```python
from build123d import *

# Parameters (mm, degrees)
F0_R     = 57.15
F0_R_2   = 27.432
F1_DEPTH = 27.94
F2_R     = 35.052
F2_R_2   = 23.495
F3_DEPTH = 5.08
F5_D     = 3.7973


with BuildPart() as f1:
    # F0 (on Top) → F1 (new body)
    with BuildSketch(Plane.XY):
        Circle(F0_R)
        Circle(F0_R_2, mode=Mode.SUBTRACT)
    extrude(amount=F1_DEPTH)

    # F2 (on face) → F3 (join)
    with BuildSketch(Plane.XY.offset(27.94)):
        Circle(F2_R)
        Circle(F2_R_2, mode=Mode.SUBTRACT)
    extrude(amount=F3_DEPTH)

    # F5 (through all)
    with Locations(Plane.XY.offset(27.94)):
        with Locations((0, -53.34), (46.1937950379, -26.67), (46.1937950379, 26.67), (0, 53.34), (-46.1937950379, 26.67), (-46.1937950379, -26.67)):
            Hole(F5_D / 2)


solid = f1.part
```
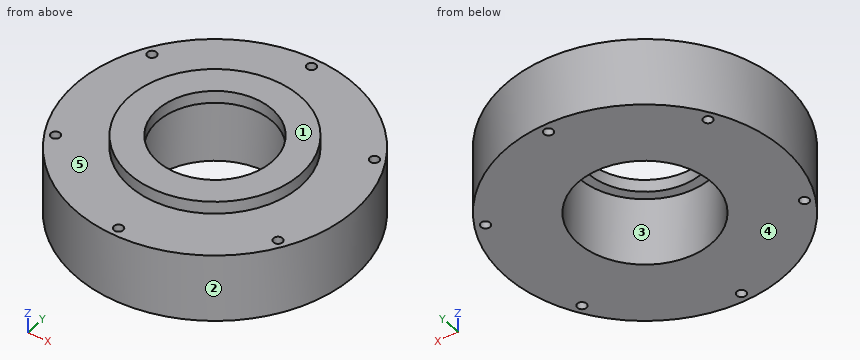
Can you work these out from the model? Positions are in its coordinate system, mm. Face numbers are marked on the shaded views. A direction names the side the tool comes from. Coordinates: 2 decimals unless noted, no trailing zeros. Loops run counter-clockwise (first coordinate to the right, second up) from the corner with the lowest first, then second, coordinate; pieces in that order, holes last.
1) Imagine slicing it at D-D on x = 15. List the corners of the cut face in (y, z) for me.
2) Thinking about a two-plate mould opening in X: for the marked faces 1, 2 and 3, which applies, pulls with the +X half, pulls with the -X half, needs draft (parallel to the pull), parting line crosses it, or undercut?
3) I need wall thicknesses on probe 1 along Y at (x, z) = (0, 19); probe 2 along Y at (x, z) = (0, 31.5) (3 decimals); probe 3 along Z at (x, y) = (-50, 22). Which ranges of each line are inside material? Lowest first, please.
4) Which directions (+Z, -Z, +X, -X, +Y, -Y) give clear straight access to the entire face, cutting with the end or side of a thin tool? Please do the marked faces 4 and 5.
5) Imagine slicing it at B-B on y = 0. List the corners of the cut face in (x, z) for me (3 decimals).
6) Imagine slicing it at A-A on x = 0. List the corners of the cut face in (y, z) for me (3 decimals), plus the area to 3 significant figures.
7) Imagine slicing it at C-C on z = 12. List the corners of the cut face in (x, y) for me.
8) For pin 1 (3 mm diameter, centred on x = 2, z = 9, fed in from -Y); pin 2 (4 mm diameter, centred on x = -32, z = 10, fed in from -Y); pin 3 (8 mm diameter, centred on x = 28.5, z = 15.5, fed in from +Y); pin 4 (2.5 mm diameter, centred on x = -46.19, y = 26.67, fed in from +Z), each with a flat end and sliding along its axis, tell me the tip position at first contact or that it passes through.
Completed:
1. outline: (-55.15, 0) - (-22.97, 0) - (-22.97, 27.94) - (-18.08, 27.94) - (-18.08, 33.02) - (-31.68, 33.02) - (-31.68, 27.94) - (-55.15, 27.94) - close; (18.08, 27.94) - (22.97, 27.94) - (22.97, 0) - (55.15, 0) - (55.15, 27.94) - (31.68, 27.94) - (31.68, 33.02) - (18.08, 33.02) - close
2. face 1: needs draft
2. face 2: parting line crosses it
2. face 3: undercut
3. probe 1: y = -57.15 to -55.24, -51.44 to -27.43, 27.43 to 51.44, 55.24 to 57.15
3. probe 2: y = -35.052 to -23.495, 23.495 to 35.052
3. probe 3: z = 0 to 27.94
4. face 4: -Z, +X, -X, +Y, -Y
4. face 5: +Z
5. outline: (-57.15, 0) - (-27.432, 0) - (-27.432, 27.94) - (-23.495, 27.94) - (-23.495, 33.02) - (-35.052, 33.02) - (-35.052, 27.94) - (-57.15, 27.94) - close; (23.495, 27.94) - (27.432, 27.94) - (27.432, 0) - (57.15, 0) - (57.15, 27.94) - (35.052, 27.94) - (35.052, 33.02) - (23.495, 33.02) - close
6. outline: (-57.15, 0) - (-55.239, 0) - (-55.239, 27.94) - (-57.15, 27.94) - close; (-51.441, 0) - (-27.432, 0) - (-27.432, 27.94) - (-23.495, 27.94) - (-23.495, 33.02) - (-35.052, 33.02) - (-35.052, 27.94) - (-51.441, 27.94) - close; (23.495, 27.94) - (27.432, 27.94) - (27.432, 0) - (51.441, 0) - (51.441, 27.94) - (35.052, 27.94) - (35.052, 33.02) - (23.495, 33.02) - close; (55.239, 0) - (57.15, 0) - (57.15, 27.94) - (55.239, 27.94) - close
6. area: 1,570 mm2
7. outline: circle Ø114.3 at (0, 0); hole circle Ø3.8 at (-46.19, -26.67); hole circle Ø3.8 at (-46.19, 26.67); hole circle Ø54.86 at (0, 0); hole circle Ø3.8 at (0, -53.34); hole circle Ø3.8 at (0, 53.34); hole circle Ø3.8 at (46.19, -26.67); hole circle Ø3.8 at (46.19, 26.67)
8. pin 1: stops at y = -57.15
8. pin 2: stops at y = -48.64
8. pin 3: stops at y = 51.63
8. pin 4: passes through
